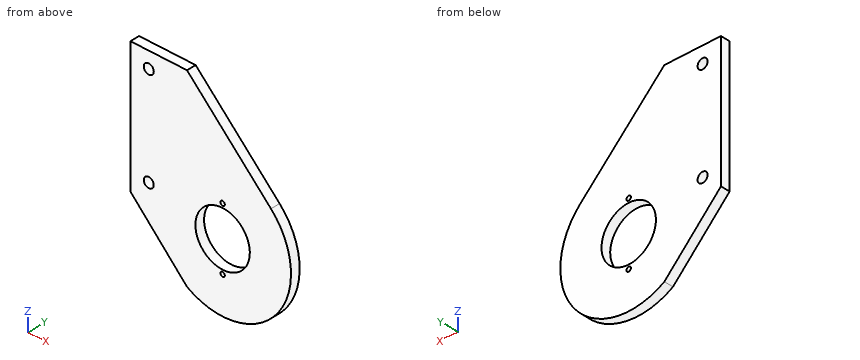
from build123d import *

# Parameters (mm, degrees)
BASE_FLANGE1_DEPTH = 6.35
SKETCH8_R          = 3.4
CUT_EXTRUDE1_DEPTH = 175.95180765
SKETCH9_R          = 18.5
CUT_EXTRUDE2_DEPTH = 175.95180765
SKETCH10_R         = 1.5
CUT_EXTRUDE3_DEPTH = 175.95180765


# Sheet-metal steps are written as plain solids
with BuildPart() as part:
    # Sketch2 → Base-Flange1 (new body)
    with BuildSketch(Plane(origin=(0, 0, 0), x_dir=(1, 0, 0), z_dir=(0, 1, 0))):
        with BuildLine():
            Line((0, 0), (38.51093065, 0))
            Line((38.51093065, 0), (95.630465325, 57.119534675))
            ThreePointArc((95.630465325, 57.119534675), (99.287953618, 118.761570635), (38.51093065, 129.682710556))
            Line((38.51093065, 129.682710556), (0, 90))
            Line((0, 90), (0, 0))
        make_face()
    extrude(amount=-BASE_FLANGE1_DEPTH)

    # Sketch8 → Cut-Extrude1 (cut, through all)
    with BuildSketch(Plane(origin=(0, 0, 0), x_dir=(1, 0, 0), z_dir=(0, 1, 0))):
        with Locations(Location((12.5, 79, 0), (0, 0, 270))):
            Circle(SKETCH8_R)
        with Locations(Location((12.5, 11, 0), (0, 0, 90))):
            Circle(SKETCH8_R)
    extrude(amount=-CUT_EXTRUDE1_DEPTH, mode=Mode.SUBTRACT)

    # Sketch9 → Cut-Extrude2 (cut, through all)
    with BuildSketch(Plane(origin=(0, 0, 0), x_dir=(1, 0, 0), z_dir=(0, 1, 0))):
        with Locations(Location((62.75, 90, 0), (0, 0, 270))):
            Circle(SKETCH9_R)
    extrude(amount=-CUT_EXTRUDE2_DEPTH, mode=Mode.SUBTRACT)

    # Sketch10 → Cut-Extrude3 (cut, through all)
    with BuildSketch(Plane(origin=(0, 0, 0), x_dir=(1, 0, 0), z_dir=(0, 1, 0))):
        with Locations(Location((62.75, 111.25, 0), (0, 0, 270))):
            Circle(SKETCH10_R)
        with Locations(Location((62.75, 68.75, 0), (0, 0, 270))):
            Circle(SKETCH10_R)
    extrude(amount=-CUT_EXTRUDE3_DEPTH, mode=Mode.SUBTRACT)


solid = part.part
Part model, mm, in its own coordinate system. Coordinates: 2 decimals unless noted, no trailing zeros. Order: outer loops, then holes, each group sorted by start corner. A loop starts at its lowest first (then second) coordinate and runs counter-clockwise, first axis right, second up.
(1) Slice it at B-B, the plane z = -111.25. Write the cut outline in (x, y).
Check sheet entries:
outline: (20.62, -6.35) - (61.25, -6.35) - (61.25, 0) - (20.62, 0) - close; (64.25, -6.35) - (104.11, -6.35) - (104.11, 0) - (64.25, 0) - close
(2) Slice it at A-A, the plane y = -1.5. Write the cut outline in (x, z), and give its area (3 significant figures).
Check sheet entries:
outline: (0, -90) - (38.51, -129.68) arc R46.5 ccw to (95.63, -57.12) - (38.51, 0) - (0, 0) - close; hole circle Ø6.8 at (12.5, -79); hole circle Ø6.8 at (12.5, -11); hole circle Ø37 at (62.75, -90); hole circle Ø3 at (62.75, -111.25); hole circle Ø3 at (62.75, -68.75)
area: 9,660 mm2
(3) Probe L1, parallel to Z at x = 59, y = -4.5; L2, parallel to X at y = -1.25, z = -98; L3, parallel to X at y = -1, z = -101. List the from-to ranges inside material, lowest first.
Check sheet entries:
L1: z = -136.35 to -108.12, -71.88 to -20.49
L2: x = 7.76 to 46.07, 79.43 to 108.56
L3: x = 10.68 to 47.88, 77.62 to 107.93
(4) Slice it at D-D, the plane x = 50. Write the cut outline in (y, z), and give its area (3 significant figures).
Check sheet entries:
outline: (-6.35, -134.72) - (0, -134.72) - (0, -103.4) - (-6.35, -103.4) - close; (-6.35, -76.6) - (0, -76.6) - (0, -11.49) - (-6.35, -11.49) - close
area: 612 mm2
(5) Slice it at C-C, the plane x = 12.5. Write the cut outline in (y, z).
Check sheet entries:
outline: (-6.35, -102.88) - (0, -102.88) - (0, -82.4) - (-6.35, -82.4) - close; (-6.35, -75.6) - (0, -75.6) - (0, -14.4) - (-6.35, -14.4) - close; (-6.35, -7.6) - (0, -7.6) - (0, 0) - (-6.35, 0) - close
(6) Pin check, flat tips, straight feed: pin 1 Ø2.5 at (x, z) = (62.75, -68.75) entering from +Y; pin 2 Ø2 at (x, y) = (84, -4) entering from -Z; pin 3 Ø3 at (y, z) = (-1.5, -117) entering from +X. Stop position of each tip, or through.
Check sheet entries:
pin 1: passes through
pin 2: stops at z = -131.86
pin 3: stops at x = 101.63
